Verification items for this drawing (mm, ordinates from the low corner). A direction names the side the tool comes from. Coordinates: 2 decimals unless noted, no trailing zeros. Write each loop counter-clockwise with the first axis right and the second up, starting at its lowest first coordinate (ties: lowest second). Pieces come first, ordered by that corner, then holes.
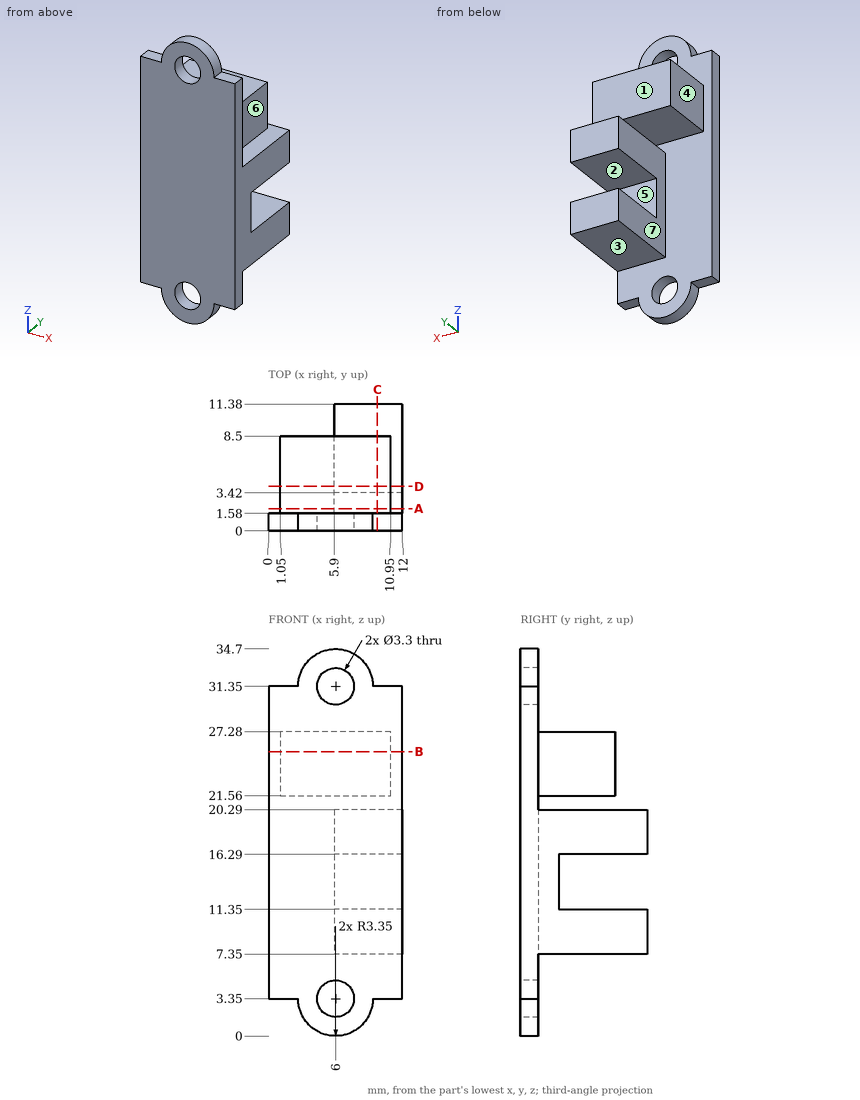
1. Thickness scan on line 1 along Z through (x, y) = (6, 0.45); line 2 along Z through (x, y) = (10.75, 2.75); line 3 along Y through (x, z) = (5.25, 22). Record the ranges inside material, lowest first.
Computed values:
line 1: z = 0 to 1.7, 5 to 29.7, 33 to 34.7
line 2: z = 7.35 to 20.29, 21.56 to 27.28
line 3: y = 0 to 8.5
2. Sectioned sample at B-B, the plane z = 25.5. Record the boundary of the cut face in (x, y), and give its area (3 significant figures).
Computed values:
outline: (0, 0) - (12, 0) - (12, 1.58) - (10.95, 1.58) - (10.95, 8.5) - (1.05, 8.5) - (1.05, 1.58) - (0, 1.58) - close
area: 87.5 mm2
3. Sectioned sample at C-C, the plane x = 9.75. Record the boundary of the cut face in (y, z), and give its area (3 significant figures).
Computed values:
outline: (0, 3.35) - (1.58, 3.35) - (1.58, 7.35) - (11.38, 7.35) - (11.38, 11.35) - (3.42, 11.35) - (3.42, 16.29) - (11.38, 16.29) - (11.38, 20.29) - (1.58, 20.29) - (1.58, 21.56) - (8.5, 21.56) - (8.5, 27.28) - (1.58, 27.28) - (1.58, 31.35) - (0, 31.35) - close
area: 171 mm2
4. Sectioned sample at D-D, the plane y = 4. Record the boundary of the cut face in (x, z).
Computed values:
outline: (1.05, 21.56) - (10.95, 21.56) - (10.95, 27.28) - (1.05, 27.28) - close; (5.9, 7.35) - (12, 7.35) - (12, 11.35) - (5.9, 11.35) - close; (5.9, 16.29) - (12, 16.29) - (12, 20.29) - (5.9, 20.29) - close
5. Sectioned sample at A-A, the plane y = 2. Record the boundary of the cut face in (x, z).
Computed values:
outline: (1.05, 21.56) - (10.95, 21.56) - (10.95, 27.28) - (1.05, 27.28) - close; (5.9, 7.35) - (12, 7.35) - (12, 20.29) - (5.9, 20.29) - close
6. Draft check along Z on the marked faces 1, 2 and 3. Enter one of: released by +Z, released by -Z, zero draft, split by the parting line, or undercut.
Computed values:
face 1: zero draft
face 2: undercut
face 3: released by -Z
7. Gauge pin test, flat ends, axial feed: pin 1 Ø1.3 at (x, y) = (11, 1) entering from +Z; pin 2 Ø5.5 at (x, y) = (4, 4.5) entering from -Z; pin 3 Ø4 at (x, z) = (6, 31.35) entering from -Y; pin 4 Ø1.5 at (x, y) = (9, 6.5) entering from +Z. Record the tip position at first contact, or that the pin passes through.
Computed values:
pin 1: stops at z = 31.35
pin 2: stops at z = 7.35
pin 3: stops at y = 0
pin 4: stops at z = 27.28
8. Access from +Z, -Z, +X, -X, +Y, -Y to the whole of each face (thin tool, end or side, straight path). Record for the marked faces 4, 5, 6 and 7.
Computed values:
face 4: +Z, -Z, -X, +Y
face 5: +X, -X, +Y
face 6: +Z, +X, +Y
face 7: -Z, -X, +Y
